from build123d import *

# Parameters (mm, degrees)
SKETCH1_W           = 500
SKETCH1_H           = 500
SKETCH1_R           = 3
BOSS_EXTRUDE1_DEPTH = 20
SKETCH2_W           = 56.144113512
SKETCH2_H           = 40.288527928
CUT_EXTRUDE2_DEPTH  = 21
SKETCH3_W           = 69.209848312
SKETCH3_H           = 67.559185152
CUT_EXTRUDE3_DEPTH  = 10
SKETCH4_R           = 2
CUT_EXTRUDE4_DEPTH  = 21


with BuildPart() as part:
    # Sketch1 → Boss-Extrude1 (new body)
    with BuildSketch(Plane(origin=(0, 0, 0), x_dir=(1, 0, 0), z_dir=(0, 1, 0))):
        Rectangle(SKETCH1_W, SKETCH1_H)
        with Locations((-128.072056756, 24.863821699)):
            Circle(SKETCH1_R, mode=Mode.SUBTRACT)
        with Locations((-71.927943244, 24.863821699)):
            Circle(SKETCH1_R, mode=Mode.SUBTRACT)
        with Locations((-71.927943244, -24.863821699)):
            Circle(SKETCH1_R, mode=Mode.SUBTRACT)
        with Locations((-128.072056756, -24.863821699)):
            Circle(SKETCH1_R, mode=Mode.SUBTRACT)
    extrude(amount=BOSS_EXTRUDE1_DEPTH)

    # Sketch2 → Cut-Extrude2 (cut, through all)
    with BuildSketch(Plane(origin=(0, 20, 0), x_dir=(1, 0, 0), z_dir=(0, 1, 0))):
        with Locations((-100, 0)):
            Rectangle(SKETCH2_W, SKETCH2_H)
    extrude(amount=-CUT_EXTRUDE2_DEPTH, mode=Mode.SUBTRACT)

    # Sketch3 → Cut-Extrude3 (cut)
    with BuildSketch(Plane.XZ):
        with Locations((-100, 0)):
            Rectangle(SKETCH3_W, SKETCH3_H)
    extrude(amount=-CUT_EXTRUDE3_DEPTH, mode=Mode.SUBTRACT)

    # Sketch4 → Cut-Extrude4 (cut, through all)
    with BuildSketch(Plane(origin=(0, 20, 0), x_dir=(1, 0, 0), z_dir=(0, 1, 0))):
        with Locations((-130.814569141, 70)):
            Circle(SKETCH4_R)
        with Locations((49.185430859, 70)):
            Circle(SKETCH4_R)
        with Locations((-40.814569141, 70)):
            Circle(SKETCH4_R)
        with Locations((-130.814569141, -70)):
            Circle(SKETCH4_R)
        with Locations((-40.814569141, -70)):
            Circle(SKETCH4_R)
        with Locations((49.185430859, -70)):
            Circle(SKETCH4_R)
        with Locations((49.185430859, 0)):
            Circle(SKETCH4_R)
        with Locations((-130.814569141, 0)):
            Circle(SKETCH4_R)
    extrude(amount=-CUT_EXTRUDE4_DEPTH, mode=Mode.SUBTRACT)


solid = part.part
Source: CAD feature listing. Evaluate the final solid. Frame: model axes, mm. Round coordinates to 2 decimals unless told otherwise and drop trailing zeros. Loops run counter-clockwise (first coordinate to the right, second up) from the corner with the lowest first, then second, coordinate; pieces in that order, holes last. Notation, with made-up numbers: M 4.5,-21 L 15.5,-21 A8 cw 15.5,-15 Z; hole C -0.5,-15.5 d10. An arc over 180 degrees is marked long. Answer as CSV lines item,"result".
Q1. Cut plane A-A (z = -10). Return the cut outline in (x, y).
Verdict:
outline,"M -250,0 L -134.6,0 L -134.6,10 L -128.07,10 L -128.07,20 L -250,20 Z; M -71.93,10 L -65.4,10 L -65.4,0 L 250,0 L 250,20 L -71.93,20 Z"
Q2. Line query: line 1 along X through (y, z) = (6.75, -70); line 2 along Z through (x, y) = (-96, 12); line 3 along X through (y, z) = (17.5, 14). Output: solid intervals per line, ascending.
Verdict:
line 1,"x = -250 to -132.81, -128.81 to -42.81, -38.81 to 47.19, 51.19 to 250"
line 2,"z = -250 to -20.14, 20.14 to 250"
line 3,"x = -250 to -128.07, -71.93 to 250"
Q3. Contact query for a flat-ended pin moving along its axis: pin 1 (9.5 mm diameter, centred on x = -128.07, z = -24.86, fed in from +Y). Output: stop coordinate, or through.
Verdict:
pin 1,"stops at y = 20"
Q4. Pull-direction query (Z, two-part tool) for faces 1 (the face through (-100, 10, -22)), 2 (the face through (-3, 0, -4)), 3 (the face through (-3, 10, 250)); classes: +Z half, -Z half, draft (parallel to the pull), parting line (faces both ways), or undercut.
Verdict:
face 1,"undercut"
face 2,"draft"
face 3,"+Z half"
